Autodesk Inventor part; units mm, degrees
ref_plane "Work Plane1" through (1.525, 0, 0) normal (0, 0, 1) x (1, 0, 0)
ref_plane "YZ Plane" through (0, 0, 0) normal (1, 0, 0) x (0, 1, 0)
ref_plane "XZ Plane" through (0, 0, 0) normal (0, 1, 0) x (-1, 0, 0)
sketch "Skizze1" plane through (0, 0, 0) normal (0, 0, 1) x (1, 0, 0)
  line L0 (0, 5.8) -> (0, 4)
  line L1 (28, 4) -> (50, 4)
  line L2 (50, 4) -> (50, 0)
  line L3 (50, 0) -> (-0.6001, 0)
  line L4 (-10.7201, 0) -> (60.12, 0)
  line L5 (-0.6001, 0) -> (-0.6001, 5.8)
  line L6 (-0.6001, 5.8) -> (0, 5.8)
  line L7 (28, 4) -> (27.2331, 4)
  line L8 (27.2331, 4) -> (0, 4)
  line L9 (0, -1.16) -> (0, 6.96)
  dimension "d0" = 50
  dimension "d1" = 22
  dimension "d2" = 8
  dimension "d9" = 0.6001
  dimension "d10" = 11.6
  dimension "d13" = 0.7669
  dimension "d14" = 8
revolve "Körper" add sketch "Skizze1" angle 360 about axis through (50, 0, 0) along (-1, 0, 0)
sketch "Skizze2" plane through (-0.6001, 0, 0) normal (-1, 0, 0) x (0, 0, 1)
  line L0 (0, 7.5056) -> (6.5, 3.7528)
  line L1 (6.5, 3.7528) -> (6.5, -3.7528)
  line L2 (6.5, -3.7528) -> (0, -7.5056)
  line L3 (0, -7.5056) -> (-6.5, -3.7528)
  line L4 (-6.5, -3.7528) -> (-6.5, 3.7528)
  line L5 (-6.5, 3.7528) -> (0, 7.5056)
  point P0 (0, 0)
  point P1 (0, 0)
  dimension "d11" = 13
extrude "Kopf" add sketch "Skizze2" along normal blind 4.7
sketch "Skizze4" plane through (0, 0, 0) normal (0, 0, 1) x (1, 0, 0)
  line L0 (-5.3001, 6.5) -> (-5.3001, 7.5056)
  line L1 (-5.3001, 7.5056) -> (-4.7195, 7.5056)
  line L2 (-4.7195, 7.5056) -> (-5.3001, 6.5)
  line L3 (-6.2401, 0) -> (0.3399, 0)
  line L4 (-0.6001, 7.5056) -> (-5.3001, 7.5056)
  line L5 (-5.3001, 3.7528) -> (-5.3001, 7.5056)
  dimension "d5" = 30
  dimension "d19" = 13
revolve "Fase1" cut sketch "Skizze4" angle 360 about axis through (-10, 0, 0) along (1, 0, 0)
thread "Gewinde"
chamfer "Fase2" distance 0.7668 distance2 0.7669 1 edges at (50, -4, 0) measured on face at (50, 1.2946, -0.3191)
ref_plane "Work Plane1" through (1.525, 0, 0) normal (0, 0, 1) x (1, 0, 0)
equation "\"d0\" = NLG"
equation "\"d1\" = GEL"
equation "\"d2\" = GD"
equation "\"d10\" = SD2"
equation "\"d14\" = BDM"
equation "\"d11\" = SW"
equation "\"d3\" = KOH - SD"
equation "\"d5\" = ANG1"
equation "\"d19\" = SW0"
equation "\"d15\" = GEL"
equation "\"d6\" = -0.5 * SPD + 0.5 * GD"
equation "\"NLG\" = 50"
equation "\"GD\" = NND"
equation "\"BDM\" = NND"
equation "\"KOH\" = 5.3"
equation "\"GEL\" = 22"
equation "\"SW\" = 13"
equation "\"SW0\" = SW"
equation "\"SPD\" = NND - 1.2269 * PTC"
equation "\"SD2\" = 11.6"
equation "\"SD\" = 0.6"
equation "\"ANG1\" = 30deg"
equation "\"GAL\" = 0.61345 * PTC"
equation "\"GUL\" = 0.61345 * PTC"
equation "\"RR\" = 0.4"
equation "\"GD1\" = THREADDIA - 1.2269 * PTC"
equation "\"THREADDIA\" = 8"
equation "\"TOA\" = 30deg"
equation "\"PTC\" = 1.25"
equation "\"NND\" = 8"
equation "\"E0\" = 1.155 * SW"
properties part number "DIN 931-1 - M8 x 50" material "Stahl, weich"
CAD build for the part. Positions are in the model's coordinates, mm. A direction names the side the tool comes from. Coordinates: 2 decimals unless noted, no trailing zeros. Loops run counter-clockwise (first coordinate to the right, second up) from the corner with the lowest first, then second, coordinate; pieces in that order, holes last. Notation, with made-up numbers: (30.25, 57.5) - (84.25, 57.5) arc R12 ccw to (84.25, 66.5) - close; hole circle Ø3 at (31, 59.5). An arc over 180 degrees is marked (long way). Write item = value, one per line. Start each with the question number.
Q1. Which spindle directions (+Z, -Z, +X, -X, +Y, -Y) get a long thin tool onto all of the face, cutting with end or side? Do faces 4 (the flat face through (-0.6, -6, -2)), 5 (the flat face through (-3, 0, 6.5)). Say none if no direction does.
Q2. Cut at A-A, the plane x = 29. List the corners of the cut face in (y, z).
Q3. Drill centre lines: L1, parallel to X at y = -6, z = 0.5; L2, parallel to Y at x = 37.5, z = -0.25; L3, parallel to X at y = -3, z = -3.5. Where is each one in solid material? Low to high.
Q4. Pull direction X, two halves, no side cores. Call faces 1 (the flat face through (0, -1.37, -3.95)), 2 (the flat face through (-5.3, 0, 0)), 3 (the cylindrical face through (24.272, -0.867, 3.905)): pulls with the +X half, pulls with the -X half, needs draft (parallel to the pull), parting line crosses it, or undercut.
Q5. Flat gauge pins, fed straight in: pin 1 Ø2 at (x, z) = (13.5, -3) entering from -Y; pin 2 Ø4 at (y, z) = (3.5, -2.5) entering from +X; pin 3 Ø1.5 at (x, z) = (36, -3) entering from -Y; pin 4 Ø1 at (y, z) = (-2.5, -4) entering from +X. Where does each tip first touch, or does it go through?
Computed:
q1.face_4 = +X
q1.face_5 = +Z, +X, -X, +Y, -Y
q2.outline = circle Ø8 at (0, 0)
q3.L1 = -5.3 to -0.6
q3.L2 = -3.99 to 3.99
q3.L3 = -5.3 to 0
q4.face_1 = pulls with the +X half
q4.face_2 = pulls with the -X half
q4.face_3 = needs draft
q5.pin_1 = -3.46
q5.pin_2 = 50
q5.pin_3 = -3.31
q5.pin_4 = 0
